Source: CAD feature listing. Evaluate the final solid. Frame: model axes, mm. A direction names the side the tool comes from. Give positions to 0.01 mm unless a question says otherwise; leave off trailing zeros. Order: outer loops, then holes, each group sorted by start corner. A loop starts at its lowest first (then second) coordinate and runs counter-clockwise, first axis right, second up.
```python
from build123d import *

# Parameters (mm, degrees)
BOSS_EXTRUDE1_DEPTH = 5
SKETCH2_W           = 20
SKETCH2_H           = 5
SKETCH2_H_2         = 6
SKETCH2_W_2         = 8
SKETCH2_H_3         = 20
SKETCH2_W_3         = 11.5
SKETCH2_H_4         = 25
SKETCH2_W_4         = 3
CUT_EXTRUDE1_DEPTH  = 10


with BuildPart() as part:
    # Sketch1 → Boss-Extrude1 (new body)
    with BuildSketch(Plane.XY):
        Polygon((6.242353031, 8.193551366), (6.242353031, 13.193551366), (-33.757646969, 13.193551366), (-33.757646969, 8.193551366), (-73.757646969, 8.193551366), (-73.757646969, 13.193551366), (-103.757646969, 13.193551366), (-103.757646969, -16.806448634), (-98.757646969, -16.806448634), (-98.757646969, -46.806448634), (-103.757646969, -46.806448634), (-103.757646969, -91.806448634), (-98.757646969, -91.806448634), (-98.757646969, -121.806448634), (-103.757646969, -121.806448634), (-103.757646969, -151.806448634), (-73.757646969, -151.806448634), (-73.757646969, -146.806448634), (-33.757646969, -146.806448634), (-33.757646969, -151.806448634), (6.242353031, -151.806448634), (6.242353031, -146.806448634), (46.242353031, -146.806448634), (46.242353031, -151.806448634), (76.242353031, -151.806448634), (76.242353031, -121.806448634), (71.242353031, -121.806448634), (71.242353031, -91.806448634), (76.242353031, -91.806448634), (76.242353031, -46.806448634), (71.242353031, -46.806448634), (71.242353031, -16.806448634), (76.242353031, -16.806448634), (76.242353031, 13.193551366), (46.242353031, 13.193551366), (46.242353031, 8.193551366), align=None)
        with BuildLine():
            ThreePointArc((21.242353031, -19.306448634), (26.242353031, -24.306448634), (21.242353031, -29.306448634))
            Line((21.242353031, -29.306448634), (6.242353031, -29.306448634))
            ThreePointArc((6.242353031, -29.306448634), (1.242353031, -24.306448634), (6.242353031, -19.306448634))
            Line((6.242353031, -19.306448634), (21.242353031, -19.306448634))
        make_face(mode=Mode.SUBTRACT)
        with BuildLine():
            Line((21.242353031, -119.306448634), (6.242353031, -119.306448634))
            ThreePointArc((6.242353031, -119.306448634), (1.242353031, -114.306448634), (6.242353031, -109.306448634))
            Line((6.242353031, -109.306448634), (21.242353031, -109.306448634))
            ThreePointArc((21.242353031, -109.306448634), (26.242353031, -114.306448634), (21.242353031, -119.306448634))
        make_face(mode=Mode.SUBTRACT)
        with BuildLine():
            Line((36.242353031, -19.306448634), (51.242353031, -19.306448634))
            ThreePointArc((51.242353031, -19.306448634), (56.242353031, -24.306448634), (51.242353031, -29.306448634))
            Line((51.242353031, -29.306448634), (36.242353031, -29.306448634))
            ThreePointArc((36.242353031, -29.306448634), (31.242353031, -24.306448634), (36.242353031, -19.306448634))
        make_face(mode=Mode.SUBTRACT)
        with BuildLine():
            ThreePointArc((51.242353031, -109.306448634), (56.242353031, -114.306448634), (51.242353031, -119.306448634))
            Line((51.242353031, -119.306448634), (36.242353031, -119.306448634))
            ThreePointArc((36.242353031, -119.306448634), (31.242353031, -114.306448634), (36.242353031, -109.306448634))
            Line((36.242353031, -109.306448634), (51.242353031, -109.306448634))
        make_face(mode=Mode.SUBTRACT)
        with BuildLine():
            Line((-53.757646969, -109.306448634), (-38.757646969, -109.306448634))
            ThreePointArc((-38.757646969, -109.306448634), (-33.757646969, -114.306448634), (-38.757646969, -119.306448634))
            Line((-38.757646969, -119.306448634), (-53.757646969, -119.306448634))
            ThreePointArc((-53.757646969, -119.306448634), (-58.757646969, -114.306448634), (-53.757646969, -109.306448634))
        make_face(mode=Mode.SUBTRACT)
        with BuildLine():
            Line((-8.757646969, -119.306448634), (-23.757646969, -119.306448634))
            ThreePointArc((-23.757646969, -119.306448634), (-28.757646969, -114.306448634), (-23.757646969, -109.306448634))
            Line((-23.757646969, -109.306448634), (-8.757646969, -109.306448634))
            ThreePointArc((-8.757646969, -109.306448634), (-3.757646969, -114.306448634), (-8.757646969, -119.306448634))
        make_face(mode=Mode.SUBTRACT)
        with BuildLine():
            Line((-53.757646969, -19.306448634), (-38.757646969, -19.306448634))
            ThreePointArc((-38.757646969, -19.306448634), (-33.757646969, -24.306448634), (-38.757646969, -29.306448634))
            Line((-38.757646969, -29.306448634), (-53.757646969, -29.306448634))
            ThreePointArc((-53.757646969, -29.306448634), (-58.757646969, -24.306448634), (-53.757646969, -19.306448634))
        make_face(mode=Mode.SUBTRACT)
        with BuildLine():
            Line((-8.757646969, -29.306448634), (-23.757646969, -29.306448634))
            ThreePointArc((-23.757646969, -29.306448634), (-28.757646969, -24.306448634), (-23.757646969, -19.306448634))
            Line((-23.757646969, -19.306448634), (-8.757646969, -19.306448634))
            ThreePointArc((-8.757646969, -19.306448634), (-3.757646969, -24.306448634), (-8.757646969, -29.306448634))
        make_face(mode=Mode.SUBTRACT)
    extrude(amount=BOSS_EXTRUDE1_DEPTH)

    # Sketch2 → Cut-Extrude1 (cut)
    with BuildSketch(Plane(origin=(0, 0, 0), x_dir=(-1, 0, 0), z_dir=(0, 0, -1))):
        with Locations((-6.242353031, -49.556448634)):
            Rectangle(SKETCH2_W, SKETCH2_H)
        with Locations((33.757646969, -49.556448634)):
            Rectangle(SKETCH2_W, SKETCH2_H)
        with Locations((33.757646969, -89.056448634)):
            Rectangle(SKETCH2_W, SKETCH2_H)
        Polygon((-16.242353031, -85.556448634), (3.757646969, -85.556448634), (9.757646969, -85.556448634), (9.757646969, -60.556448634), (-21.242353031, -60.556448634), (-21.242353031, -85.556448634), align=None)
        with Locations((-6.242353031, -88.556448634)):
            Rectangle(SKETCH2_W, SKETCH2_H_2)
        with Locations((49.757646969, -69.306448634)):
            Rectangle(SKETCH2_W_2, SKETCH2_H_3)
        with Locations((-29.992353031, -73.056448634)):
            Rectangle(SKETCH2_W_3, SKETCH2_H_4)
        with Locations((-22.742353031, -73.056448634)):
            Rectangle(SKETCH2_W_4, SKETCH2_H_4)
    extrude(amount=-CUT_EXTRUDE1_DEPTH, mode=Mode.SUBTRACT)


solid = part.part
```
1) Draft query along X for faces 6 (the flat face through (-46, -109.306, 2)), 7 (the flat face through (61, -151.806, 2)), 8 (the flat face through (26, -85.556, 2)), 9 (the flat face through (71.242, -107, 2)). Return one class per face: +X half, -X half, draft (parallel to the pull), parting line (faces both ways), or undercut.
Report:
face 6: undercut
face 7: draft
face 8: undercut
face 9: +X half
2) Reachability of faces 1 (the flat face through (-101, -91.806, 2)), 2 (the flat face through (-89, 13.194, 2)), 3 (the flat face through (27, 8.194, 2)), 4 (the flat face through (-73.758, -149, 2)), 5 (the flat face through (-34, -47.056, 2)) from +Z, -Z, +X, -X, +Y, -Y: full face, straight path, thin tool, end or side. Return the list, or none.
Report:
face 1: +Z, -Z, -X
face 2: +Z, -Z, +X, -X, +Y
face 3: +Z, -Z, +Y
face 4: +Z, -Z, -Y
face 5: +Z, -Z
3) Section query C-C, the plane x = 43.5. Return the cut outline in (y, z).
Report:
outline: (-146.81, 0) - (-119.31, 0) - (-119.31, 5) - (-146.81, 5) - close; (-109.31, 0) - (-29.31, 0) - (-29.31, 5) - (-109.31, 5) - close; (-19.31, 0) - (8.19, 0) - (8.19, 5) - (-19.31, 5) - close
4) Material intervals for L1, parallel to Y at x = 0, z = 4.3; L2, parallel to Y at x = 6, z = 2.95; L3, parallel to Y at x = 50.5, z = 0.45, sorted ascending.
Report:
L1: y = -151.81 to -91.56, -60.56 to -52.06, -47.06 to 13.19
L2: y = -151.81 to -119.3, -109.31 to -91.56, -60.56 to -52.06, -47.06 to -29.3, -19.31 to 13.19
L3: y = -151.81 to -119.31, -109.31 to -29.31, -19.31 to 13.19
5) Section query D-D, the plane z = 3.55. Count the separate pieces of the cut face and the enclosed holes in it, and give its area (3 significant figures).
Report:
separate pieces: 1
enclosed holes: 13
area: 24,800 mm2
6) Section query B-B, the plane x = -50.5. Return the cut outline in (y, z), and give its area (3 significant figures).
Report:
outline: (-146.81, 0) - (-119.31, 0) - (-119.31, 5) - (-146.81, 5) - close; (-109.31, 0) - (-79.31, 0) - (-79.31, 5) - (-109.31, 5) - close; (-59.31, 0) - (-29.31, 0) - (-29.31, 5) - (-59.31, 5) - close; (-19.31, 0) - (8.19, 0) - (8.19, 5) - (-19.31, 5) - close
area: 575 mm2
7) Pin query (flat end, axial travel): pin 1 (1.5 mm diameter, centred on x = -37.5, z = 2.5, fed in from -Y); pin 2 (1.5 mm diameter, centred on x = 45, z = 3.5, fed in from +Y). Return the tip coordinate at first contact, or that it passes through.
Report:
pin 1: stops at y = -146.81
pin 2: stops at y = 8.19
8) Section query A-A, the plane x = -18.5. Return the cut outline in (y, z), and give its area (3 significant figures).
Report:
outline: (-151.81, 0) - (-119.31, 0) - (-119.31, 5) - (-151.81, 5) - close; (-109.31, 0) - (-29.31, 0) - (-29.31, 5) - (-109.31, 5) - close; (-19.31, 0) - (13.19, 0) - (13.19, 5) - (-19.31, 5) - close
area: 725 mm2
